```python
from build123d import *

# Parameters (mm, degrees)
F0_W     = 723.9
F0_H     = 330.2
F1_DEPTH = 19.05
F2_SIZE  = 12.7
F3_D     = 25.4


with BuildPart() as f1:
    # F0 (on Top) → F1 (new body)
    with BuildSketch(Plane.XY):
        with Locations((33.9713070929, -3.6599552712)):
            Rectangle(F0_W, F0_H)
    extrude(amount=F1_DEPTH)

    # F2
    f2_edges = [f1.edges().sort_by_distance(p)[0] for p in [
        (395.921307, -3.659955, 19.05),
        (-327.978693, -3.659955, 19.05),
        (33.971307, -168.759955, 19.05),
    ]]
    chamfer(f2_edges, length=F2_SIZE)

    # F3 (through all)
    with Locations(Plane(origin=(0, 0, 0), x_dir=(1, 0, 0), z_dir=(0, 0, -1))):
        with Locations((-277.1786929071, -110.6400447288)):
            Hole(F3_D / 2)


solid = f1.part
```
Here's how the part is built. I have some questions about the finished solid (model axes, mm). Give positions to 0.01 mm unless a question says otherwise; leave off trailing zeros. Write each loop counter-clockwise with the first axis right and the second up, starting at its lowest first coordinate (ties: lowest second). Pieces come first, ordered by that corner, then holes.
(1) Will these pins go through, and if not, where does the flat tip stop? pin 1 (8 mm diameter, centred on x = 193.5, z = 13.5, fed in from -Y); pin 2 (1.5 mm diameter, centred on y = 31.5, z = 11.5, fed in from -X); pin 3 (5 mm diameter, centred on x = 254.5, z = 14.5, fed in from -Y).
Output values:
pin 1: stops at y = -165.61
pin 2: stops at x = -323.58
pin 3: stops at y = -163.11
(2) Thinking about a two-plate mould opening in Y: for faces 1 (the face through (29, -1, 0)), 2 (the face through (29, 161.44, 9)), 3 (the face through (-264.49, 110.08, 9.66)), 4 (the face through (28.9, -162.32, 12.79)), which applies, pulls with the +Y half, pulls with the -Y half, needs draft (parallel to the pull), parting line crosses it, or undercut?
Output values:
face 1: needs draft
face 2: pulls with the +Y half
face 3: undercut
face 4: pulls with the -Y half
(3) If I drill on L1, parallel to X at y = 3, z = 6.5; L2, parallel to Y at x = -279.5, z = 1.75; L3, parallel to X at y = -77.5, z = 14.25, over which ranges is the centre line in solid material (lowest first)?
Output values:
L1: x = -327.83 to 395.77
L2: y = -168.76 to 98.15, 123.13 to 161.44
L3: x = -320.08 to 388.02
(4) Imagine slicing it at A-A, the plane z = 16. Write out the boundary of the cut face in (x, y).
Output values:
outline: (-318.33, -159.11) - (386.27, -159.11) - (386.27, 161.44) - (-318.33, 161.44) - close; hole circle Ø25.4 at (-277.18, 110.64)
